Geometry check sheet. Reference: the model listing, model coordinates, mm. Face numbers are marked on the shaded views. A direction names the side the tool comes from. Give positions to 0.01 mm unless a question says otherwise; leave off trailing zeros. Loops run counter-clockwise (first coordinate to the right, second up) from the corner with the lowest first, then second, coordinate; pieces in that order, holes last.
1. Tool access check on the marked faces 1 and 2. Record the directions out of +Z, -Z, +X, -X, +Y, -Y that give a thin tool (end or side, any length) a straight path to the whole face; none if there is none.
2. Material ranges on L1, parallel to Y at x = 441, z = 1500; L2, parallel to Z at x = 431, y = -1; L3, parallel to Z at x = 395, y = 43.5, recorded low to high.
3. Cross-section at A-A, the plane z = 146. Record the cut outline in (x, y), plus the area to 3 significant figures.
4. Cross-section at C-C, the plane x = 227. Record the cut outline in (y, z).
5. Cross-section at D-D, the plane z = 922. Record the cut outline in (x, y), plus the area to 3 significant figures.
6. Go/stop test with flat-tipped pins: pin 1 Ø8 at (y, z) = (-100, 1355.5) entering from -X; pin 2 Ø5 at (x, z) = (83.5, 231) entering from +Y; pin 3 Ø1.5 at (x, y) = (351, -99.5) entering from -Z. Record where each tip stops, or that it passes through.
7. Cross-section at B-B, the plane y = 93.5. Record the cut outline in (x, z), plus the area to 3 significant figures.
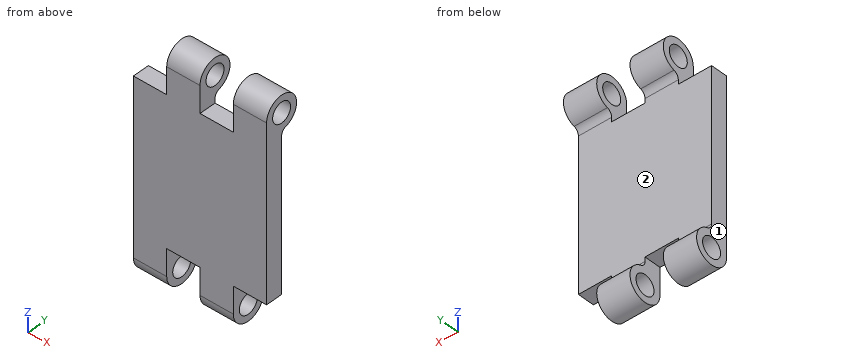
from build123d import *

# Parameters (mm, degrees)
BOSS_EXTRUDE1_DEPTH     = 500
BOSS_EXTRUDE2_START     = 250
SKETCH1_3_R             = 125
SKETCH1_3_R_2           = 75
BOSS_EXTRUDE2_DEPTH     = 250
SKETCH1_4_R             = 125
SKETCH1_4_R_2           = 75
BOSS_EXTRUDE3_DEPTH     = 250
BOSS_EXTRUDE4_START     = -250
SKETCH1_5_R             = 125
SKETCH1_5_R_2           = 75
BOSS_EXTRUDE4_DEPTH     = 250
BOSS_EXTRUDE5_START     = 500
SKETCH1_6_R             = 125
SKETCH1_6_R_2           = 75
BOSS_EXTRUDE5_DEPTH     = 250
CUT_EXTRUDE1_DEPTH      = 250
CUT_EXTRUDE1_DEPTH_BACK = 250
FILLET1_R               = 50


with BuildPart() as part:
    # Sketch1 → Boss-Extrude1 (new, symmetric)
    with BuildSketch(Plane(origin=(0, 0, 0), x_dir=(0, 0, -1), z_dir=(1, 0, 0))):
        with BuildLine():
            ThreePointArc((0, -125), (-88.388347648, -88.388347648), (-125, 0))
            Line((-125, 0), (-1375, 0))
            ThreePointArc((-1375, 0), (-1411.611652352, -88.388347648), (-1500, -125))
            Line((-1500, -125), (0, -125))
        make_face()
    extrude(amount=BOSS_EXTRUDE1_DEPTH, both=True)

    # Sketch1_3 → Boss-Extrude2 (add)
    with BuildSketch(Plane(origin=(0, 0, 0), x_dir=(0, 0, -1), z_dir=(1, 0, 0)).offset(BOSS_EXTRUDE2_START)):
        Circle(SKETCH1_3_R)
        Circle(SKETCH1_3_R_2, mode=Mode.SUBTRACT)
    extrude(amount=-BOSS_EXTRUDE2_DEPTH)

    # Sketch1_4 → Boss-Extrude3 (add)
    with BuildSketch(Plane(origin=(0, 0, 0), x_dir=(0, 0, -1), z_dir=(1, 0, 0))):
        with Locations((-1500, 0)):
            Circle(SKETCH1_4_R)
        with Locations((-1500, 0)):
            Circle(SKETCH1_4_R_2, mode=Mode.SUBTRACT)
    extrude(amount=-BOSS_EXTRUDE3_DEPTH)

    # Sketch1_5 → Boss-Extrude4 (add)
    with BuildSketch(Plane(origin=(0, 0, 0), x_dir=(0, 0, -1), z_dir=(1, 0, 0)).offset(BOSS_EXTRUDE4_START)):
        Circle(SKETCH1_5_R)
        Circle(SKETCH1_5_R_2, mode=Mode.SUBTRACT)
    extrude(amount=-BOSS_EXTRUDE4_DEPTH)

    # Sketch1_6 → Boss-Extrude5 (add)
    with BuildSketch(Plane(origin=(0, 0, 0), x_dir=(0, 0, -1), z_dir=(1, 0, 0)).offset(BOSS_EXTRUDE5_START)):
        with Locations((-1500, 0)):
            Circle(SKETCH1_6_R)
        with Locations((-1500, 0)):
            Circle(SKETCH1_6_R_2, mode=Mode.SUBTRACT)
    extrude(amount=-BOSS_EXTRUDE5_DEPTH)

    # Sketch2 → Cut-Extrude1 (cut, two sides: drawn at the far end of the back side and taken through both)
    with BuildSketch(Plane(origin=(0, 0, 0), x_dir=(1, 0, 0), z_dir=(0, 1, 0)).offset(-CUT_EXTRUDE1_DEPTH_BACK)):
        Polygon((-250, 550.682417094), (-250, -200), (0, -200), (0, 342.970708342), (250, 342.970708342), (250, -200), (760.214276003, -200), (760.214276003, 550.682417094), align=None)
        Polygon((250, -2214.630516483), (250, -1300), (0, -1300), (0, -1946.053133522), (-250, -1946.053133522), (-250, -1300), (-708.69599817, -1300), (-708.69599817, -2214.630516483), align=None)
    extrude(amount=CUT_EXTRUDE1_DEPTH + CUT_EXTRUDE1_DEPTH_BACK, mode=Mode.SUBTRACT)

    # Fillet1
    fillet1_edges = [part.edges().sort_by_distance(p)[0] for p in [
        (125, 0, 125),
        (-125, 0, 1375),
        (-375, 0, 125),
        (375, 0, 1375),
    ]]
    fillet(fillet1_edges, radius=FILLET1_R)


solid = part.part
Result:
1. face 1: +Z, -Z, -X, +Y, -Y
1. face 2: +X, -X, +Y
2. L1: y = -125 to -75, 75 to 125
2. L2: z = 200 to 1425.01, 1574.99 to 1625
2. L3: z = 1382.81 to 1438.9, 1561.1 to 1617.19
3. outline: (-500, -125) - (-250, -125) - (-250, 4.96) - (-500, 4.96) - close; (0, -125) - (250, -125) - (250, 4.96) - (0, 4.96) - close
3. area: 65,000 mm2
4. outline: (-125, 0) arc R125 ccw (long way) to (35.71, 119.79) arc R50 cw to (0, 167.71) - (0, 1300) - (-125, 1300) - close; hole circle Ø150 at (0, 0)
5. outline: (-500, -125) - (500, -125) - (500, 0) - (-500, 0) - close
5. area: 125,000 mm2
6. pin 1: stops at x = -250
6. pin 2: stops at y = 0
6. pin 3: stops at z = 200
7. outline: (-500, -82.96) - (-250, -82.96) - (-250, 82.96) - (-500, 82.96) - close; (-250, 1417.04) - (0, 1417.04) - (0, 1582.96) - (-250, 1582.96) - close; (0, -82.96) - (250, -82.96) - (250, 82.96) - (0, 82.96) - close; (250, 1417.04) - (500, 1417.04) - (500, 1582.96) - (250, 1582.96) - close
7. area: 166,000 mm2
